Source: CAD feature listing. Evaluate the final solid. Frame: model axes, mm. Give positions to 0.01 mm unless a question says otherwise; leave off trailing zeros. Order: outer loops, then holes, each group sorted by start corner. A loop starts at its lowest first (then second) coordinate and runs counter-clockwise, first axis right, second up. Notation, with made-up numbers: (47, 60) -> (92, 60) arc R28 cw to (92, 79) -> close; hole circle Ø5 at (73.25, -9). An arc over 180 degrees is marked (long way). Answer in a Markdown table with one row per item.
```python
from build123d import *

# Parameters (mm, degrees)
SKETCH1_R           = 2.4257
BOSS_EXTRUDE1_DEPTH = 3.175
FILLET1_R           = 3.175
SKETCH2_R           = 4.3688
CUT_EXTRUDE1_DEPTH  = 153.961206275


with BuildPart() as part:
    # Sketch1 → Boss-Extrude1 (new body)
    with BuildSketch(Plane(origin=(0, 0, 0), x_dir=(1, 0, 0), z_dir=(0, 1, 0))):
        Polygon((0, 0), (0, 114.3), (38.1, 114.3), (101.6, 38.1), (101.6, 0), align=None)
        with Locations(Location((15.875, 15.875, 0), (0, 0, 270))):
            Circle(SKETCH1_R, mode=Mode.SUBTRACT)
        with Locations(Location((53.975, 15.875, 0), (0, 0, 270))):
            Circle(SKETCH1_R, mode=Mode.SUBTRACT)
        with Locations(Location((92.075, 15.875, 0), (0, 0, 270))):
            Circle(SKETCH1_R, mode=Mode.SUBTRACT)
        with Locations(Location((16.891, 53.975, 0), (0, 0, 270))):
            Circle(SKETCH1_R, mode=Mode.SUBTRACT)
        with Locations(Location((16.891, 79.375, 0), (0, 0, 270))):
            Circle(SKETCH1_R, mode=Mode.SUBTRACT)
        with Locations(Location((16.891, 104.775, 0), (0, 0, 270))):
            Circle(SKETCH1_R, mode=Mode.SUBTRACT)
    extrude(amount=BOSS_EXTRUDE1_DEPTH)

    # Fillet1
    fillet1_edges = [part.edges().sort_by_distance(p)[0] for p in [
        (0, 1.5875, 0),
        (0, 1.5875, -114.3),
        (38.1, 1.5875, -114.3),
        (101.6, 1.5875, -38.1),
        (101.6, 1.5875, 0),
    ]]
    fillet(fillet1_edges, radius=FILLET1_R)

    # Sketch2 → Cut-Extrude1 (cut, through all)
    with BuildSketch(Plane.XZ):
        with Locations(Location((50.8, -50.8, 0), (0, 0, 270))):
            Circle(SKETCH2_R)
    extrude(amount=-CUT_EXTRUDE1_DEPTH, mode=Mode.SUBTRACT)


solid = part.part
```
(1) Section query C-C (x = 64). Return the cut outline in (y, z) (3 decimals).
A:
| item | result |
|---|---|
| outline | (0, -83.22) -> (3.175, -83.22) -> (3.175, 0) -> (0, 0) -> close |
(2) Ray query, probe 1 along Z at (x, y) = (53, 1.6); probe 2 along Z at (x, y) = (16, 2.7); probe 3 along X at (y, z) = (2.75, -103). Return the intervals inside material, ascending.
A:
| item | result |
|---|---|
| probe 1 | z = -96.42 to -54.57, -47.03 to -18.1, -13.65 to 0 |
| probe 2 | z = -114.3 to -107.03, -102.52 to -81.63, -77.12 to -56.23, -51.72 to -18.3, -13.45 to 0 |
| probe 3 | x = 0 to 15.24, 18.54 to 47.52 |
(3) Pull-direction query (X, two-part tool) for faces 1 (the cylindrical face through (16.6, 1.57, -13.56)), 2 (the flat face through (20, 2, -114.3)), 3 (the cylindrical face through (17.62, 1.57, -51.66)), 4 (the cylindrical face through (0.91, 1.61, -0.95)); classes: +X half, -X half, draft (parallel to the pull), parting line (faces both ways), or undercut.
A:
| item | result |
|---|---|
| face 1 | undercut |
| face 2 | draft |
| face 3 | undercut |
| face 4 | -X half |
(4) Section query A-A (z = -48.5). Return the cut outline in (x, y) (3 decimals), plus the area to 3 significant figures.
A:
| item | result |
|---|---|
| outline | (0, 0) -> (47.086, 0) -> (47.086, 3.175) -> (0, 3.175) -> close; (54.514, 0) -> (92.933, 0) -> (92.933, 3.175) -> (54.514, 3.175) -> close |
| area | 271 mm^2 |
(5) Section query D-D (z = -93.5). Return the cut outline in (x, y) (3 decimals).
A:
| item | result |
|---|---|
| outline | (0, 0) -> (55.433, 0) -> (55.433, 3.175) -> (0, 3.175) -> close |
(6) Section query B-B (y = 1.2). Give the number of separate pieces and of enclosed holes in the cut face, plus the area to 3 significant figures.
A:
| item | result |
|---|---|
| separate pieces | 1 |
| enclosed holes | 7 |
| area | 9,020 mm^2 |
(7) First-contact query: pin 1 Ø6.5 at (x, z) = (16.891, -104.775) entering from -Y; pin 2 Ø4 at (x, z) = (53.975, -15.875) entering from -Y; pin 3 Ø1.5 at (y, z) = (1, -62) entering from +X. Flat tips, straight axial feed; report the tip coordinate or a pass-through.
A:
| item | result |
|---|---|
| pin 1 | stops at y = 0 |
| pin 2 | passes through |
| pin 3 | stops at x = 82.31 |
